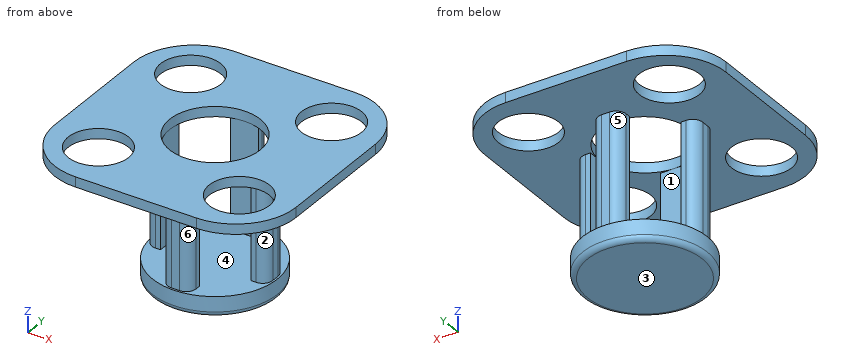
from build123d import *

# Parameters (mm, degrees)
SKETCH2_R           = 3
BOSS_EXTRUDE2_DEPTH = 1
SKETCH6_W           = 1.4
SKETCH6_H           = 1.5
SKETCH6_W_2         = 1.5
SKETCH6_H_2         = 1.4
BOSS_EXTRUDE5_DEPTH = 11
FILLET4_R           = 1
SKETCH8_R           = 4.5
CUT_EXTRUDE1_DEPTH  = 20
SKETCH9_R           = 6.2
BOSS_EXTRUDE6_DEPTH = 2
FILLET5_R           = 0.5


with BuildPart() as part:
    # Sketch2 → Boss-Extrude2 (new body)
    with BuildSketch(Plane.XY):
        with BuildLine():
            Line((-12, 0), (-12, 6))
            ThreePointArc((-12, 6), (-10.242640687, 10.242640687), (-6, 12))
            Line((-6, 12), (0, 12))
            Line((0, 12), (6, 12))
            ThreePointArc((6, 12), (10.242640687, 10.242640687), (12, 6))
            Line((12, 6), (12, 0))
            Line((12, 0), (12, -6))
            ThreePointArc((12, -6), (10.242640687, -10.242640687), (6, -12))
            Line((6, -12), (0, -12))
            Line((0, -12), (-6, -12))
            ThreePointArc((-6, -12), (-10.242640687, -10.242640687), (-12, -6))
            Line((-12, -6), (-12, 0))
        make_face()
        with Locations((7, 7)):
            Circle(SKETCH2_R, mode=Mode.SUBTRACT)
        with Locations((-7, 7)):
            Circle(SKETCH2_R, mode=Mode.SUBTRACT)
        with Locations((-7, -7)):
            Circle(SKETCH2_R, mode=Mode.SUBTRACT)
        with Locations((7, -7)):
            Circle(SKETCH2_R, mode=Mode.SUBTRACT)
        Circle(SKETCH2_R, mode=Mode.SUBTRACT)
    extrude(amount=BOSS_EXTRUDE2_DEPTH)

    # Sketch6 → Boss-Extrude5 (add)
    with BuildSketch(Plane(origin=(0, 0, 0), x_dir=(-1, 0, 0), z_dir=(0, 0, -1))):
        with Locations((-0.7, -5.25)):
            Rectangle(SKETCH6_W, SKETCH6_H)
        with Locations((0.7, -5.25)):
            Rectangle(SKETCH6_W, SKETCH6_H)
        Polygon((4.5, -1.4), (4.5, 0), (4.5, 1.4), (6, 1.4), (6, -1.4), align=None)
        with Locations((0.7, 5.25)):
            Rectangle(SKETCH6_W, SKETCH6_H)
        with Locations((-0.7, 5.25)):
            Rectangle(SKETCH6_W, SKETCH6_H)
        with Locations((-5.25, -0.7)):
            Rectangle(SKETCH6_W_2, SKETCH6_H_2)
        with Locations((-5.25, 0.7)):
            Rectangle(SKETCH6_W_2, SKETCH6_H_2)
    extrude(amount=BOSS_EXTRUDE5_DEPTH)

    # Fillet4
    fillet4_edges = [part.edges().sort_by_distance(p)[0] for p in [
        (1.4, -6, -5.5),
        (-1.4, -6, -5.5),
        (-6, -1.4, -5.5),
        (-6, 1.4, -5.5),
        (-1.4, 6, -5.5),
        (1.4, 6, -5.5),
        (6, 1.4, -5.5),
        (6, -1.4, -5.5),
    ]]
    fillet(fillet4_edges, radius=FILLET4_R)

    # Sketch8 → Cut-Extrude1 (cut)
    with BuildSketch(Plane(origin=(0, 0, -11), x_dir=(-1, 0, 0), z_dir=(0, 0, -1))):
        with Locations(Location((0, 0, 0), (0, 0, 180))):
            Circle(SKETCH8_R)
    extrude(amount=-CUT_EXTRUDE1_DEPTH, mode=Mode.SUBTRACT)

    # Sketch9 → Boss-Extrude6 (add)
    with BuildSketch(Plane(origin=(0, 0, -11), x_dir=(-1, 0, 0), z_dir=(0, 0, -1))):
        Circle(SKETCH9_R)
    extrude(amount=BOSS_EXTRUDE6_DEPTH)

    # Fillet5
    fillet5_edges = [part.edges().sort_by_distance(p)[0] for p in [
        (6.2, 0, -13),
    ]]
    fillet(fillet5_edges, radius=FILLET5_R)


solid = part.part
CAD build for the part. Positions are in the model's coordinates, mm. Face numbers are marked on the shaded views. A direction names the side the tool comes from. Give positions to 0.01 mm unless a question says otherwise; leave off trailing zeros. Order: outer loops, then holes, each group sorted by start corner. A loop starts at its lowest first (then second) coordinate and runs counter-clockwise, first axis right, second up. Notation, with made-up numbers: (-7, -17) -> (52, -17) arc R29 ccw to (52, 5) -> close; hole circle Ø11 at (40, 50.5). An arc over 180 degrees is marked (long way). Return JSON: item names as keys, results as strings.
Q1. Saw through at D-D (x = 10.75). Write the cut outline in (y, z).
Working result:
{"outline": "(-9.67, 0) -> (9.67, 0) -> (9.67, 1) -> (-9.67, 1) -> close"}
Q2. Saw through at A-A (z = -9). Write the cut outline in (x, y).
Working result:
{"outline": "(-6, -0.4) arc R1 ccw to (-5, -1.4) -> (-4.5, -1.4) -> (-4.5, 1.4) -> (-5, 1.4) arc R1 ccw to (-6, 0.4) -> close; (-1.4, -5) arc R1 ccw to (-0.4, -6) -> (0.4, -6) arc R1 ccw to (1.4, -5) -> (1.4, -4.5) -> (-1.4, -4.5) -> close; (-1.4, 4.5) -> (1.4, 4.5) -> (1.4, 5) arc R1 ccw to (0.4, 6) -> (-0.4, 6) arc R1 ccw to (-1.4, 5) -> close; (4.5, -1.4) -> (5, -1.4) arc R1 ccw to (6, -0.4) -> (6, 0.4) arc R1 ccw to (5, 1.4) -> (4.5, 1.4) -> close"}
Q3. Which spindle directions (+Z, -Z, +X, -X, +Y, -Y) get a long thin tool onto all of the face, cutting with end or side? Do the marked faces 4, 5 and 6. Say none if no direction does.
Working result:
{"face 4": "none", "face 5": "-X, +Y", "face 6": "+X, -Y"}
Q4. Drill centre lines: line 1 (Y direction, x = 0, z = 0.65); line 2 (Z direction, x = -0.75, y = 8.5); line 3 (Y direction, x = 7, z = 0.85). Where is each one in solid material? Low to high.
Working result:
{"line 1": "-12 to -4.5, 4.5 to 12", "line 2": "0 to 1", "line 3": "-11.92 to -10, -4 to 4, 10 to 11.92"}
Q5. Flat gauge pins, fed straight in: pin 1 (1.4 mm diameter, centred on y = 0.5, z = -7.5, fed in from +X); pin 2 (0.8 mm diameter, centred on x = 0.5, z = -3.5, fed in from +Y); pin 3 (0.6 mm diameter, centred on x = -4.5, z = -3, fed in from -Y); pin 4 (5 mm diameter, centred on x = 7, y = -7, fed in from -Z). Where does each tip first touch, or does it go through?
Working result:
{"pin 1": "x = 6", "pin 2": "y = 6", "pin 3": "y = -1.4", "pin 4": "through"}
Q6. Saw through at B-B (x = 7). Write the cut outline in (y, z), then the cut area to 3 significant figures.
Working result:
{"outline": "(-11.92, 0) -> (-10, 0) -> (-10, 1) -> (-11.92, 1) -> close; (-4, 0) -> (4, 0) -> (4, 1) -> (-4, 1) -> close; (10, 0) -> (11.92, 0) -> (11.92, 1) -> (10, 1) -> close", "area": "11.8 mm²"}
Q7. Mould opens along Y. For the marked faces 1, 2 and 3 say: pulls with the +Y half, pulls with the -Y half, needs draft (parallel to the pull), parting line crosses it, or undercut.
Working result:
{"face 1": "undercut", "face 2": "pulls with the -Y half", "face 3": "needs draft"}
